Can you work these out from the drawing? Everything is in mm from the part's minimum corner. A direction names the side the tool comes from. Round coordinates to 2 decimals unless told otherwise and drop trailing zeros. Write each loop counter-clockwise with the first axis right and the second up, starting at its lowest first coordinate (ties: lowest second). Pieces come first, ordered by that corner, then holes.
Q1. We'd pull the mould along X, two halves only. Please class the marked faces 1, 2 and 3: +X half, -X half, draft (parallel to the pull), parting line (faces both ways), or undercut.
Q2. I'm going to push flat-ended pins straight in: pin 1 Ø5 at (y, z) = (18, 6.5) entering from +X; pin 2 Ø1.5 at (x, y) = (10.5, 16) entering from -Z; pin 3 Ø4 at (x, y) = (3.5, 6.5) entering from -Z. Where does each tip first touch, or does it pass through?
Q3. For the marked faces 4 and 5, which set-ups out of +Z, -Z, +X, -X, +Y, -Y let a thin tool reach every point of the face, with its end or its side?
Q4. If we section it at A-A (z = 12.5): Please give me the cut outline in (x, y).
Q5. If we section it at D-D (y = 18.75): Please give me the cut outline in (x, z), plus the area to 3 significant figures.
Q6. If we section it at C-C (y = 2.5): Please give me the cut outline in (x, z), plus the area to 3 significant figures.
Q7. Please list where these lines run through material, in increasing order: line 1 along Z through (x, y) = (12.5, 7.5); line 2 along Y through (x, z) = (10.5, 22.75); line 3 along Z through (x, y) = (10, 6.25).
Q8. If we section it at B-B (x = 12.5): Please give me the cut outline in (y, z).
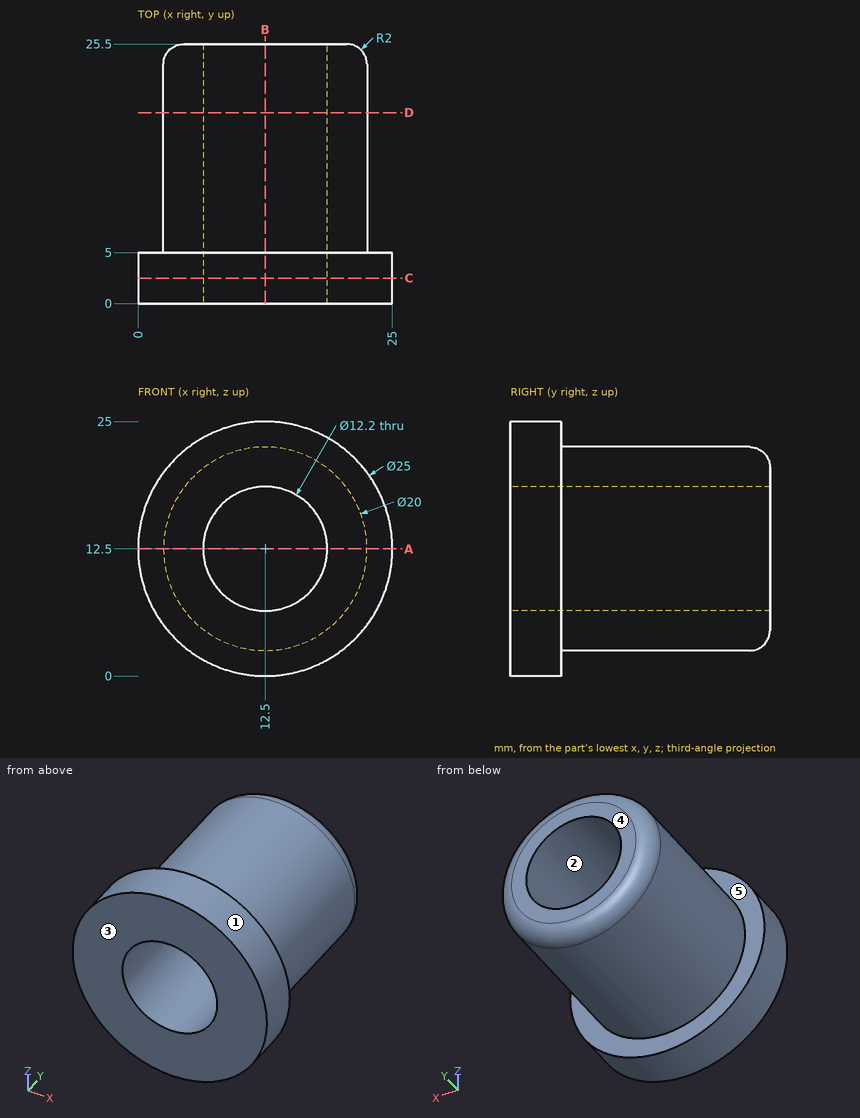
A:
1. face 1: parting line
1. face 2: undercut
1. face 3: draft
2. pin 1: stops at x = 21.87
2. pin 2: stops at z = 2.58
2. pin 3: stops at z = 2.64
3. face 4: +Z, -Z, +X, -X, +Y
3. face 5: +Y
4. outline: (0, 0) - (6.4, 0) - (6.4, 25.5) - (4.5, 25.5) arc R2 ccw to (2.5, 23.5) - (2.5, 5) - (0, 5) - close; (18.6, 0) - (25, 0) - (25, 5) - (22.5, 5) - (22.5, 23.5) arc R2 ccw to (20.5, 25.5) - (18.6, 25.5) - close
5. outline: circle Ø20 at (12.5, 12.5); hole circle Ø12.2 at (12.5, 12.5)
5. area: 197 mm2
6. outline: circle Ø25 at (12.5, 12.5); hole circle Ø12.2 at (12.5, 12.5)
6. area: 374 mm2
7. line 1: z = 2.5 to 6.4, 18.6 to 22.5
7. line 2: y = 0 to 5
7. line 3: z = 2.82 to 6.94, 18.06 to 22.18
8. outline: (0, 0) - (5, 0) - (5, 2.5) - (23.5, 2.5) arc R2 ccw to (25.5, 4.5) - (25.5, 6.4) - (0, 6.4) - close; (0, 18.6) - (25.5, 18.6) - (25.5, 20.5) arc R2 ccw to (23.5, 22.5) - (5, 22.5) - (5, 25) - (0, 25) - close
